Could you check a few things on this model? Use its own coordinates, in mm. A direction names the side the tool comes from. Give positions to 0.01 mm unless a question says otherwise; leave off trailing zeros. Loops run counter-clockwise (first coordinate to the right, second up) from the corner with the lowest first, then second, coordinate; pieces in that order, holes last. Notation, with made-up numbers: (32, -1) - (55, -1) arc R18 ccw to (55, 12) - close; hole circle Ø5 at (47, -35). An arc over 180 degrees is marked (long way). One line per item, written item: value. Start each with the question number.
Q1. I'm going to push flat-ended pins straight in: P1, Ø18, axis at x = 54.5, z = 20, coming from the +Y side; P2, Ø3, axis at x = -44, y = 6.5, coming from the +Z side; P3, Ø3, axis at y = -3.5, z = 60, coming from the +X side. Where does each tip first touch, or does it pass through?
Q2. If I drill on line 1 (X direction, y = 19.25, z = 64); line 2 (X direction, y = 18.5, z = 23.5); line 3 (Z direction, x = -2.5, y = -11.5), over which ranges is the centre line in solid material (lowest first)? Write a range as from..to.
Q3. I want a section at B-B (z = 42.5). Please give me the cut outline in (x, y), then the cut area to 3 significant figures.
Q4. For faces 1 (the face through (-23.953, 17.015, 74.395)), 2 (the face through (65, 20, 46)), 3 (the face through (-34.305, -8, 71)), 4 (the face through (98, -9.981, 41)), which set-ups out of +Z, -Z, +X, -X, +Y, -Y let a thin tool reach every point of the face, with its end or its side?
Q5. If we mould it in two halves opening along X, with no side actions, what happens to faces 5 (the face through (47.7, 0.8, 0)), 6 (the face through (115.695, 42, 40)), 7 (the face through (-23.953, 17.015, 7.395)), 8 (the face through (-66.5, -7.6, 1.71))? For each: released by +X, released by -X, zero draft, split by the parting line, or undercut.
Q6. I want a section at C-C (z = 64). Please give me the cut outline in (x, y).
Q7. I want a section at D-D (x = -21). Please give me the cut outline in (y, z).
Q8. I want a section at A-A (x = 71). Please give me the cut outline in (y, z).
```python
from build123d import *

# Parameters (mm, degrees)
BOSS_EXTRUDE1_DEPTH = 82
SKETCH2_W           = 66
SKETCH2_H           = 50
CUT_EXTRUDE1_DEPTH  = 36
SKETCH3_R           = 10
CUT_EXTRUDE2_DEPTH  = 36
BOSS_EXTRUDE6_DEPTH = 39
SKETCH5_R           = 7.2
CUT_EXTRUDE3_DEPTH  = 27
REVOLVE2_ANGLE      = 180
CUT_EXTRUDE4_DEPTH  = 153
SKETCH10_W          = 54
SKETCH10_H          = 36
CUT_EXTRUDE5_DEPTH  = 17
SKETCH11_W          = 17
SKETCH11_H          = 36
CUT_REVOLVE2_ANGLE  = 180
FILLET1_R           = 4
FILLET2_R           = 6


with BuildPart() as part:
    # Sketch1 → Boss-Extrude1 (new body)
    with BuildSketch(Plane.XY):
        Polygon((-68.304856892, -15.980758971), (115.695143108, -15.980758971), (115.695143108, 46.019241029), (73.695143108, 46.019241029), (73.695143108, 1.019241029), (-68.304856892, 1.019241029), align=None)
    extrude(amount=BOSS_EXTRUDE1_DEPTH)

    # Sketch2 → Cut-Extrude1 (cut)
    with BuildSketch(Plane(origin=(115.695143108, 0, 0), x_dir=(0, 0, -1), z_dir=(1, 0, 0))):
        with Locations((-41, 15.019241029)):
            Rectangle(SKETCH2_W, SKETCH2_H)
    extrude(amount=-CUT_EXTRUDE1_DEPTH, mode=Mode.SUBTRACT)

    # Sketch3 → Cut-Extrude2 (cut)
    with BuildSketch(Plane(origin=(0, 0, 0), x_dir=(-1, 0, 0), z_dir=(0, 0, -1))):
        with Locations((-97.695143108, 27.019241029)):
            Circle(SKETCH3_R)
    extrude(amount=-CUT_EXTRUDE2_DEPTH, mode=Mode.SUBTRACT)

    # Sketch4 → Boss-Extrude6 (add)
    with BuildSketch(Plane(origin=(0, 1.019241029, 0), x_dir=(1, 0, 0), z_dir=(0, 1, 0))):
        with BuildLine():
            Line((55.695143108, -46), (73.695143108, -46))
            Line((73.695143108, -46), (73.695143108, -82))
            Line((73.695143108, -82), (55.695143108, -82))
            ThreePointArc((55.695143108, -82), (37.695143108, -64), (55.695143108, -46))
        make_face()
    boss_extrude6 = extrude(amount=BOSS_EXTRUDE6_DEPTH)

    # Sketch5 → Cut-Extrude3 (cut)
    with BuildSketch(Plane(origin=(0, 40.019241029, 0), x_dir=(1, 0, 0), z_dir=(0, 1, 0))):
        with Locations(Location((55.695143108, -64, 0), (0, 0, 270))):
            Circle(SKETCH5_R)
    cut_extrude3 = extrude(amount=-CUT_EXTRUDE3_DEPTH, mode=Mode.SUBTRACT)

    # Mirror3: Boss-Extrude6, Cut-Extrude3 across plane
    add(boss_extrude6.mirror(Plane.XY.offset(41)))
    add(cut_extrude3.mirror(Plane.XY.offset(41)), mode=Mode.SUBTRACT)

    # Sketch7 → Revolve2 (revolve)
    with BuildSketch(Plane(origin=(0, 1.019241029, 0), x_dir=(1, 0, 0), z_dir=(0, 1, 0))):
        Polygon((-24.304856892, 0), (-24.304856892, -82), (-8.304856892, -82), (-8.304856892, -67), (10.695143108, -67), (10.695143108, -15), (-8.304856892, -15), (-8.304856892, 0), align=None)
    revolve(axis=Axis((-24.304856892, 1.019241029, 0), (0, 0, 1)), revolution_arc=REVOLVE2_ANGLE)

    # Sketch8 → Cut-Extrude4 (cut)
    with BuildSketch(Plane.XY.offset(82)):
        with BuildLine():
            Line((-14.304856892, 1.019241029), (-14.304856892, -15.980758971))
            Line((-14.304856892, -15.980758971), (-34.304856892, -15.980758971))
            Line((-34.304856892, -15.980758971), (-34.304856892, 1.019241029))
            ThreePointArc((-34.304856892, 1.019241029), (-24.304856892, 11.019241029), (-14.304856892, 1.019241029))
        make_face()
    extrude(amount=-CUT_EXTRUDE4_DEPTH, mode=Mode.SUBTRACT)

    # Sketch10 → Cut-Extrude5 (cut)
    with BuildSketch(Plane.XZ.offset(15.980758971)):
        with Locations((-24.304856892, 41)):
            Rectangle(SKETCH10_W, SKETCH10_H)
    extrude(amount=-CUT_EXTRUDE5_DEPTH, mode=Mode.SUBTRACT)

    # Sketch11 → Cut-Revolve2 (revolve, cut)
    with BuildSketch(Plane.XZ.offset(-1.019241029)):
        with Locations((-5.804856892, 41)):
            Rectangle(SKETCH11_W, SKETCH11_H)
    revolve(axis=Axis((-24.304856892, 1.019241029, 0), (0, 0, 1)), revolution_arc=CUT_REVOLVE2_ANGLE, mode=Mode.SUBTRACT)

    # Fillet1
    fillet1_edges = [part.edges().sort_by_distance(p)[0] for p in [
        (79.695143108, 15.019241029, 74),
        (79.695143108, 15.019241029, 8),
    ]]
    fillet(fillet1_edges, radius=FILLET1_R)

    # Fillet2
    fillet2_edges = [part.edges().sort_by_distance(p)[0] for p in [
        (73.695143108, 43.019241029, 82),
        (-68.304856892, -7.480758971, 82),
        (73.695143108, 43.019241029, 0),
        (-68.304856892, -7.480758971, 0),
    ]]
    fillet(fillet2_edges, radius=FILLET2_R)


solid = part.part
```
Worked answers:
1. P1: stops at y = 40.02
1. P2: stops at z = 67
1. P3: stops at x = 79.7
2. line 1: x = -54.18..5.57, 37.7..48.5, 62.9..79.7
2. line 2: x = -54.63..-44.88, -3.73..6.02, 38.56..51.05, 60.34..79.7
2. line 3: z = 0..23, 59..82
3. outline: (-68.3, -15.98) - (-51.3, -15.98) - (-51.3, 1.02) arc R27 cw to (2.7, 1.02) - (2.7, -15.98) - (115.7, -15.98) - (115.7, -9.98) - (79.7, -9.98) - (79.7, 40.02) - (115.7, 40.02) - (115.7, 46.02) - (73.7, 46.02) - (73.7, 1.02) - (10.7, 1.02) arc R35 ccw to (-59.3, 1.02) - (-68.3, 1.02) - close
3. area: 3,080 mm²
4. face 1: +Z, +Y
4. face 2: +Y
4. face 3: +Z, -Z, -Y
4. face 4: +X
5. face 5: zero draft
5. face 6: released by +X
5. face 7: undercut
5. face 8: released by -X
6. outline: (-68.3, -15.98) - (-34.3, -15.98) - (-34.3, 1.02) arc R10 cw to (-14.3, 1.02) - (-14.3, -15.98) - (115.7, -15.98) - (115.7, -9.98) - (79.7, -9.98) - (79.7, 40.02) - (115.7, 40.02) - (115.7, 46.02) - (73.7, 46.02) - (73.7, 40.02) - (62.9, 40.02) - (62.9, 13.02) - (48.5, 13.02) - (48.5, 40.02) - (37.7, 40.02) - (37.7, 1.02) - (10.7, 1.02) arc R35 ccw to (-59.3, 1.02) - (-68.3, 1.02) - close
7. outline: (10.46, 0) - (16.67, 0) - (16.67, 15) - (35.86, 15) - (35.86, 67) - (16.67, 67) - (16.67, 82) - (10.46, 82) - (10.46, 59) - (27.82, 59) - (27.82, 23) - (10.46, 23) - close
8. outline: (-15.98, 0) - (40.02, 0) - (40.02, 36) - (1.02, 36) - (1.02, 46) - (40.02, 46) - (40.02, 82) - (-15.98, 82) - close
